Verification items for the finished model (mm, model axes). Face numbers are marked on the shaded views. A direction names the side the tool comes from. Give positions to 0.01 mm unless a question says otherwise; leave off trailing zeros. Loops run counter-clockwise (first coordinate to the right, second up) from the corner with the lowest first, then second, coordinate; pieces in that order, holes last. Notation, with made-up numbers: (-28.75, -40) - (29.25, -40) arc R34 cw to (29.25, -9) - close; hole circle Ø1 at (86, 4.25). An arc over 180 degrees is marked (long way). One line per question, with ' | ' between items. Start each with the question number.
1. Mould release check, pull along X, two halves, no side actions. Record for the marked faces 5, 6 and 7: +X half, -X half, draft (parallel to the pull), parting line (faces both ways), or undercut.
2. Section check B-B, the plane x = -25. Enter the section's corners in (y, z).
3. Section check D-D, the plane x = 8.5. Enter the section's corners in (y, z).
4. Depth check by flat-ended pin: pin 1 Ø10 at (y, z) = (-10.5, 16) entering from +X; pin 2 Ø4 at (x, z) = (21.5, 9) entering from +Y; pin 3 Ø1.2 at (x, z) = (11, -1) entering from -Y; pin 4 Ø3 at (x, y) = (40.65, -17.2) entering from +Z. Enter the tip coordinate at first touch or a pass-through.
5. Tool access check on the marked faces 1, 2, 3 and 4. Record the directions out of +Z, -Z, +X, -X, +Y, -Y that give a thin tool (end or side, any length) a straight path to the whole face; none if there is none.
6. Section check A-A, the plane x = -40.65. Enter the section's corners in (y, z), then the cut area to 3 significant figures.
7. Thickness scan on line 1 along Y through (x, z) = (40.65, -0.5); line 2 along Z through (x, y) = (7, 4); line 3 along Y through (x, z) = (-10, 5.75). Record the ranges inside material, lowest first. Write a range as from..to.
from build123d import *
from build123d.topology import SkipClean

# Parameters (mm, degrees)
CROQUIS1_W              = 87
CROQUIS1_H              = 27
SALIENTE_EXTRUIR1_DEPTH = 12.5
CROQUIS2_R              = 2
CROQUIS2_W              = 87.3
CROQUIS2_H              = 28.4
CROQUIS2_W_2            = 87
CROQUIS2_H_2            = 27
SALIENTE_EXTRUIR3_DEPTH = 1.5
CROQUIS3_R              = 6.5
SALIENTE_EXTRUIR4_DEPTH = 3
CROQUIS4_R              = 7.5
SALIENTE_EXTRUIR5_DEPTH = 1.4
CROQUIS8_W              = 21
CROQUIS8_H              = 15
CORTAR_EXTRUIR2_DEPTH   = 0.1
SALIENTE_EXTRUIR6_DEPTH = 1.7


with BuildPart() as part:
    # Croquis1 → Saliente-Extruir1 (new body)
    with BuildSketch(Plane.XY):
        Rectangle(CROQUIS1_W, CROQUIS1_H)
    extrude(amount=SALIENTE_EXTRUIR1_DEPTH)

    # Croquis2 → Saliente-Extruir3 (add)
    # profile 1 of 6: a face of its own
    with BuildSketch(Plane(origin=(0, 0, 0), x_dir=(-1, 0, 0), z_dir=(0, 0, -1))):
        with BuildLine():
            Line((37.65, 14.2), (43.65, 14.2))
            Line((43.65, 14.2), (43.65, 17.2))
            ThreePointArc((43.65, 17.2), (40.65, 20.2), (37.65, 17.2))
            Line((37.65, 17.2), (37.65, 14.2))
        make_face()
        with Locations((40.65, 17.2)):
            Circle(CROQUIS2_R, mode=Mode.SUBTRACT)
    # profile 2 of 6: a face of its own
    with BuildSketch(Plane(origin=(0, 0, 0), x_dir=(-1, 0, 0), z_dir=(0, 0, -1))):
        with BuildLine():
            Line((43.65, -17.2), (43.65, -14.2))
            Line((43.65, -14.2), (37.65, -14.2))
            Line((37.65, -14.2), (37.65, -17.2))
            ThreePointArc((37.65, -17.2), (40.65, -20.2), (43.65, -17.2))
        make_face()
        with Locations((40.65, -17.2)):
            Circle(CROQUIS2_R, mode=Mode.SUBTRACT)
    # profile 3 of 6: a face of its own
    with BuildSketch(Plane(origin=(0, 0, 0), x_dir=(-1, 0, 0), z_dir=(0, 0, -1))):
        with BuildLine():
            Line((-37.65, -17.2), (-37.65, -14.2))
            Line((-37.65, -14.2), (-43.65, -14.2))
            Line((-43.65, -14.2), (-43.65, -17.2))
            ThreePointArc((-43.65, -17.2), (-40.65, -20.2), (-37.65, -17.2))
        make_face()
        with Locations((-40.65, -17.2)):
            Circle(CROQUIS2_R, mode=Mode.SUBTRACT)
    # profile 4 of 6: a face of its own
    with BuildSketch(Plane(origin=(0, 0, 0), x_dir=(-1, 0, 0), z_dir=(0, 0, -1))):
        with BuildLine():
            Line((-43.65, 14.2), (-37.65, 14.2))
            Line((-37.65, 14.2), (-37.65, 17.2))
            ThreePointArc((-37.65, 17.2), (-40.65, 20.2), (-43.65, 17.2))
            Line((-43.65, 17.2), (-43.65, 14.2))
        make_face()
        with Locations((-40.65, 17.2)):
            Circle(CROQUIS2_R, mode=Mode.SUBTRACT)
    # profile 5 of 6: a face of its own
    with BuildSketch(Plane(origin=(0, 0, 0), x_dir=(-1, 0, 0), z_dir=(0, 0, -1))):
        Rectangle(CROQUIS2_W, CROQUIS2_H)
        Rectangle(CROQUIS2_W_2, CROQUIS2_H_2, mode=Mode.SUBTRACT)
    # profile 6 of 6: a face of its own
    with BuildSketch(Plane(origin=(0, 0, 0), x_dir=(-1, 0, 0), z_dir=(0, 0, -1))):
        Rectangle(CROQUIS2_W_2, CROQUIS2_H_2)
    extrude(amount=SALIENTE_EXTRUIR3_DEPTH)

    # Croquis3 → Saliente-Extruir4 (add)
    with BuildSketch(Plane.XY.offset(12.5)):
        with Locations((8.5, 0)):
            Circle(CROQUIS3_R)
    extrude(amount=SALIENTE_EXTRUIR4_DEPTH)

    # Croquis4 → Saliente-Extruir5 (add)
    with BuildSketch(Plane.XY.offset(15.5)):
        with Locations((8.5, 0)):
            Circle(CROQUIS4_R)
    extrude(amount=SALIENTE_EXTRUIR5_DEPTH)

    # Croquis7 → Revoluci_n3 (revolve)
    with SkipClean():  # the faces are left unmerged after this step: merging them gives an invalid solid
        with BuildSketch(Plane(origin=(0, 0, 0), x_dir=(1, 0, 0), z_dir=(0, 1, 0))):
            with BuildLine():
                Line((8.5, -16.9), (2.5, -16.9))
                ThreePointArc((2.5, -16.9), (5.407670781, -18.019316877), (8.5, -18.4))
                Line((8.5, -18.4), (8.5, -16.9))
            make_face()
            with BuildLine():
                Line((14.5, -16.9), (8.5, -16.9))
                Line((8.5, -16.9), (8.5, -18.4))
                ThreePointArc((8.5, -18.4), (11.592329219, -18.019316877), (14.5, -16.9))
            make_face()
        revolve(axis=Axis((8.5, 0, 16.9), (0, 0, 1)))
    add(part.part.scale(1), mode=Mode.REPLACE)  # the faces are merged on a copy

    # Croquis8 → Cortar-Extruir2 (cut)
    with BuildSketch(Plane.XY.offset(12.5)):
        with Locations((28.15, 0)):
            Rectangle(CROQUIS8_W, CROQUIS8_H)
    extrude(amount=-CORTAR_EXTRUIR2_DEPTH, mode=Mode.SUBTRACT)

    # Croquis9 → Saliente-Extruir6 (add)
    # profile 1 of 2: a face of its own
    with BuildSketch(Plane.ZY.offset(43.5)):
        with BuildLine():
            Line((0, -3.25), (0, 3.25))
            ThreePointArc((0, 3.25), (1.75, 5), (3.5, 3.25))
            Line((3.5, 3.25), (3.5, -3.25))
            ThreePointArc((3.5, -3.25), (1.75, -5), (0, -3.25))
        make_face()
        with BuildLine():
            Line((0.3, -3.25), (0.3, 3.25))
            ThreePointArc((0.3, 3.25), (1.75, 4.7), (3.2, 3.25))
            Line((3.2, 3.25), (3.2, -3.25))
            ThreePointArc((3.2, -3.25), (1.75, -4.7), (0.3, -3.25))
        make_face(mode=Mode.SUBTRACT)
    # profile 2 of 2: a face of its own
    with BuildSketch(Plane.ZY.offset(43.5)):
        with BuildLine():
            Line((1.5, -3.25), (1.5, 3.25))
            ThreePointArc((1.5, 3.25), (1.75, 3.5), (2, 3.25))
            Line((2, 3.25), (2, -3.25))
            ThreePointArc((2, -3.25), (1.75, -3.5), (1.5, -3.25))
        make_face()
    extrude(amount=SALIENTE_EXTRUIR6_DEPTH)


solid = part.part
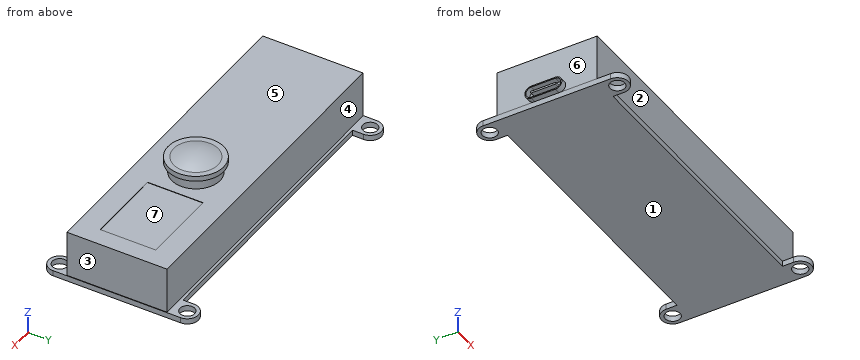
Results list:
1) face 5: draft | face 6: -X half | face 7: undercut
2) outline: (-14.2, -1.5) - (14.2, -1.5) - (14.2, 0) - (13.5, 0) - (13.5, 12.5) - (-13.5, 12.5) - (-13.5, 0) - (-14.2, 0) - close
3) outline: (-14.2, -1.5) - (14.2, -1.5) - (14.2, 0) - (13.5, 0) - (13.5, 12.5) - (6.5, 12.5) - (6.5, 15.5) - (7.5, 15.5) - (7.5, 16.9) - (6, 16.9) arc R12.75 ccw to (-6, 16.9) - (-7.5, 16.9) - (-7.5, 15.5) - (-6.5, 15.5) - (-6.5, 12.5) - (-13.5, 12.5) - (-13.5, 0) - (-14.2, 0) - close
4) pin 1: x = 43.5 | pin 2: y = 13.5 | pin 3: y = -14.2 | pin 4: through
5) face 1: -Z, +X, -X, +Y, -Y | face 2: +Z, +X, -X, -Y | face 3: +Z, +X, +Y, -Y | face 4: +Z, +X, -X, +Y
6) outline: (-20.2, -1.5) - (-19.2, -1.5) - (-19.2, 0) - (-20.2, 0) - close; (-15.2, -1.5) - (15.2, -1.5) - (15.2, 0) - (13.5, 0) - (13.5, 12.5) - (-13.5, 12.5) - (-13.5, 0) - (-15.2, 0) - close; (19.2, -1.5) - (20.2, -1.5) - (20.2, 0) - (19.2, 0) - close | area: 386 mm²
7) line 1: -20.2..-19.2, -15.2..15.2, 19.2..20.2 | line 2: -1.5..17.66 | line 3: -13.5..13.5
